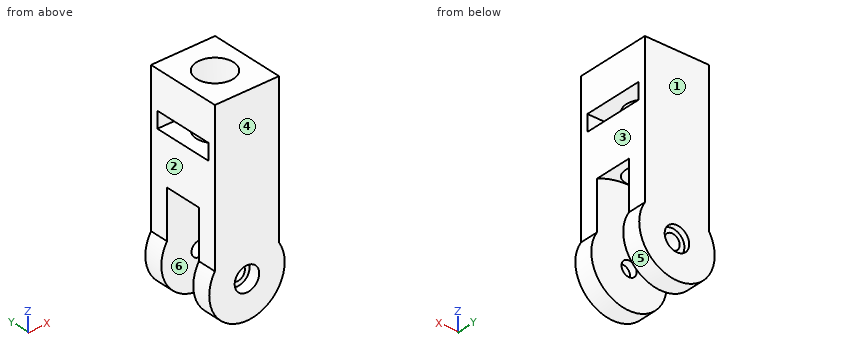
```python
from build123d import *

# Parameters (mm, degrees)
SKETCH_1_W               = 17
SKETCH_1_H               = 20
EXTRUDE_1_DEPTH          = 40
SKETCH_3_R               = 10
SKETCH_3_R_2             = 2
EXTRUDE_2_DEPTH          = 10
EXTRUDE_START            = -5
SKETCH_4_R               = 10
SKETCH_4_R_2             = 2
EXTRUDE_3_DEPTH          = 5
SKETCH_5_R               = 20
CUT_EXTRUDE_1_DEPTH      = 10
CUT_EXTRUDE_2_REACH      = 66.858
CUT_EXTRUDE_2_END_RADIUS = 20
SKETCH_6_R               = 4.9
CUT_EXTRUDE_3_REACH      = 53.865
SKETCH_7_W               = 4.3
SKETCH_7_H               = 16
SKETCH_8_R               = 3.25
CUT_EXTRUDE_4_DEPTH      = 3
CUT_EXTRUDE_START        = -1.5
SKETCH_9_R               = 3.25
CUT_EXTRUDE_5_DEPTH      = 1.5


with BuildPart() as part:
    # 草图1 → 凸台-拉伸1 (new body)
    with BuildSketch(Plane.XY):
        with Locations((-10.828446216, -17.343796091)):
            Rectangle(SKETCH_1_W, SKETCH_1_H)
    extrude(amount=EXTRUDE_1_DEPTH)

    # 草图3 → 凸台-拉伸2 (add)
    with BuildSketch(Plane.XZ.offset(27.343796091)):
        with Locations((-10.828446216, -5)):
            Circle(SKETCH_3_R)
        with Locations(Location((-10.828446216, -5, 0), (0, 0, 270))):
            Circle(SKETCH_3_R_2, mode=Mode.SUBTRACT)
    extrude(amount=-EXTRUDE_2_DEPTH)

    # 草图4 → 凸台-拉伸3 (add)
    with BuildSketch(Plane(origin=(0, -7.343796091, 0), x_dir=(1, 0, 0), z_dir=(0, 1, 0)).offset(EXTRUDE_START)):
        with Locations((-10.828446216, 5)):
            Circle(SKETCH_4_R)
        with Locations(Location((-10.828446216, 5, 0), (0, 0, 90))):
            Circle(SKETCH_4_R_2, mode=Mode.SUBTRACT)
    extrude(amount=EXTRUDE_3_DEPTH)

    # 草图5 → 切除-拉伸1 (cut)
    with BuildSketch(Plane.XZ.offset(12.343796091)):
        with Locations((-10.828446216, -5)):
            Circle(SKETCH_5_R)
    extrude(amount=CUT_EXTRUDE_1_DEPTH, mode=Mode.SUBTRACT)

    # 切除-拉伸2: up to this cylinder (the profile starts outside it)
    cut_extrude_2_end = Plane(origin=(-10.828446216, -17.343796, -5), z_dir=(0, 1, 0)) * Cylinder(CUT_EXTRUDE_2_END_RADIUS, 174.716, mode=Mode.PRIVATE)
    # 草图6 → 切除-拉伸2 (cut, up to the surface)
    with BuildSketch(Plane.XY.offset(40), mode=Mode.PRIVATE) as cut_extrude_2_sk1:
        with Locations((-10.828446216, -17.343796091)):
            Circle(SKETCH_6_R)
    cut_extrude_2_tool1 = extrude(cut_extrude_2_sk1.sketch, amount=-CUT_EXTRUDE_2_REACH, mode=Mode.PRIVATE) - cut_extrude_2_end
    add(cut_extrude_2_tool1.solids().sort_by_distance((-10.828446, -17.343796, 40))[0], mode=Mode.SUBTRACT)

    # 草图7 → 切除-拉伸3 (cut, up to next)
    with BuildSketch(Plane(origin=(-2.328446216, 0, 0), x_dir=(0, 0, -1), z_dir=(1, 0, 0)), mode=Mode.PRIVATE) as cut_extrude_3_sk1:
        with Locations((-27.85, -17.343796091)):
            Rectangle(SKETCH_7_W, SKETCH_7_H)
    cut_extrude_3_tool1 = extrude(cut_extrude_3_sk1.sketch, amount=-CUT_EXTRUDE_3_REACH, mode=Mode.PRIVATE) & part.part
    add(cut_extrude_3_tool1.solids().sort_by_distance((-2.328446, -17.343796, 27.85))[0], mode=Mode.SUBTRACT)

    # 草图8 → 切除-拉伸4 (cut)
    with BuildSketch(Plane.XZ.offset(27.343796091)):
        with Locations(Location((-10.828446216, -5, 0), (0, 0, 270))):
            Circle(SKETCH_8_R)
    extrude(amount=-CUT_EXTRUDE_4_DEPTH, mode=Mode.SUBTRACT)

    # 草图9 → 切除-拉伸5 (cut)
    with BuildSketch(Plane(origin=(0, -7.343796091, 0), x_dir=(1, 0, 0), z_dir=(0, 1, 0)).offset(CUT_EXTRUDE_START)):
        with Locations(Location((-10.828446216, 5, 0), (0, 0, 90))):
            Circle(SKETCH_9_R)
    extrude(amount=CUT_EXTRUDE_5_DEPTH, mode=Mode.SUBTRACT)


solid = part.part
```
CAD build for the part. Positions are in the model's coordinates, mm. Face numbers are marked on the shaded views. A direction names the side the tool comes from. Coordinates: 2 decimals unless noted, no trailing zeros. Write each loop counter-clockwise with the first axis right and the second up, starting at its lowest first coordinate (ties: lowest second). Pieces come first, ordered by that corner, then holes.
(1) 3-axis set-ups, long thin cutter, end or side, ignore diameter. For the marked faces 1, 2 and 3: which of +Z, -Z, +X, -X, +Y, -Y reach the whole face in a straight line?
(2) Cut at B-B, the plane y = -10.5. List the corners of the cut face in (x, z), and give its area (3 significant figures).
(3) Flat gauge pins, fed straight in: pin 1 (10 mm diameter, centred on y = -13.5, z = 3.5, fed in from +X); pin 2 (5 mm diameter, centred on x = -12.5, y = -20, fed in from -Z); pin 3 (3 mm diameter, centred on y = -18, z = 15, fed in from -X). Where does each tip first touch, or does it go through?
(4) Cut at C-C, the plane x = -13.5. List the corners of the cut face in (y, z), and give its area (3 significant figures).
(5) Two-plate mould, pull along Y, no slides. Class the marked faces 4, 5 and 6: +Y half, -Y half, draft (parallel to the pull), parting line (faces both ways), or undercut.
(6) Cut at D-D, the plane y = -20.75. List the corners of the cut face in (x, z).
(7) Drill centre lines: probe 1 along Y at (x, z) = (-11.5, -11); probe 2 along X at (y, z) = (-8.5, -5); probe 3 along Y at (x, z) = (-13, 28). Where is each one in solid material? Low to high.
(8) Cut at A-A, the plane z = -5. List the corners of the cut face in (x, y), and give its area (3 significant figures).
Geometry says:
1. face 1: +Z, -Z, +X, -X, +Y
1. face 2: +Z, -X, +Y, -Y
1. face 3: +Z, +X, +Y, -Y
2. outline: (-19.33, 0.27) arc R10 ccw (long way) to (-2.33, 0.27) - (-2.33, 25.7) - (-19.33, 25.7) - close; (-19.33, 30) - (-2.33, 30) - (-2.33, 40) - (-19.33, 40) - close; hole circle Ø4 at (-10.83, -5)
2. area: 847 mm2
3. pin 1: stops at x = -1.51
3. pin 2: stops at z = -14.97
3. pin 3: stops at x = -19.33
4. outline: (-27.34, -14.64) - (-22.34, -14.64) - (-22.34, 14.82) - (-21.45, 14.82) - (-21.45, 25.7) - (-25.34, 25.7) - (-25.34, 30) - (-21.45, 30) - (-21.45, 40) - (-27.34, 40) - (-27.34, -3.15) - (-24.34, -3.15) - (-24.34, -6.85) - (-27.34, -6.85) - close; (-13.24, 14.82) - (-12.34, 14.82) - (-12.34, -14.64) - (-7.34, -14.64) - (-7.34, -6.85) - (-8.84, -6.85) - (-8.84, -3.15) - (-7.34, -3.15) - (-7.34, 40) - (-13.24, 40) - (-13.24, 30) - (-9.34, 30) - (-9.34, 25.7) - (-13.24, 25.7) - close
4. area: 541 mm2
5. face 4: -Y half
5. face 5: draft
5. face 6: undercut
6. outline: (-19.33, 13.1) arc R20 cw to (-14.35, 14.69) - (-14.35, 25.7) - (-19.33, 25.7) - close; (-19.33, 30) - (-14.35, 30) - (-14.35, 40) - (-19.33, 40) - close; (-7.31, 14.69) arc R20 cw to (-2.33, 13.1) - (-2.33, 25.7) - (-7.31, 25.7) - close; (-7.31, 30) - (-2.33, 30) - (-2.33, 40) - (-7.31, 40) - close
7. probe 1: y = -27.34 to -22.34, -12.34 to -7.34
7. probe 2: x = -20.83 to -14.08, -7.58 to -0.83
7. probe 3: y = -27.34 to -25.34, -9.34 to -7.34
8. outline: (-20.83, -27.34) - (-14.08, -27.34) - (-14.08, -24.34) - (-12.83, -24.34) - (-12.83, -22.34) - (-20.83, -22.34) - close; (-20.83, -12.34) - (-12.83, -12.34) - (-12.83, -8.84) - (-14.08, -8.84) - (-14.08, -7.34) - (-20.83, -7.34) - close; (-8.83, -24.34) - (-7.58, -24.34) - (-7.58, -27.34) - (-0.83, -27.34) - (-0.83, -22.34) - (-8.83, -22.34) - close; (-8.83, -12.34) - (-0.83, -12.34) - (-0.83, -7.34) - (-7.58, -7.34) - (-7.58, -8.84) - (-8.83, -8.84) - close
8. area: 149 mm2
